Part model, mm, in its own coordinate system. A direction names the side the tool comes from. Give positions to 0.01 mm unless a question says otherwise; leave off trailing zeros. Loops run counter-clockwise (first coordinate to the right, second up) from the corner with the lowest first, then second, coordinate; pieces in that order, holes last. Notation, with made-up numbers: M -9.75,60 L 6.25,60 A14 cw 6.25,65 Z; hole C 27,-38 d6. An arc over 180 degrees is marked long. Answer in a Markdown table with one row per item.
from build123d import *

# Parameters (mm, degrees)
BOSS_EXTRUDE1_DEPTH = 20
SHELL1_T            = -2
BOSS_EXTRUDE2_START = 1
SKETCH2_R           = 50
BOSS_EXTRUDE2_DEPTH = 1
SKETCH3_R           = 2.5
CUT_EXTRUDE1_DEPTH  = 96.067235106
CIRPATTERN1_COUNT   = 3


with BuildPart() as part:
    # Sketch1 → Boss-Extrude1 (new body)
    with BuildSketch(Plane(origin=(0, 0, 0), x_dir=(1, 0, 0), z_dir=(0, 1, 0))):
        with BuildLine():
            Line((-31.353657468, -234.344603511), (-21.203657468, -216.764287814))
            Line((-21.203657468, -216.764287814), (-37.324683077, -207.456809339))
            ThreePointArc((-37.324683077, -207.456809339), (0, -190.726435625), (37.324683077, -207.456809339))
            Line((37.324683077, -207.456809339), (21.203657468, -216.764287814))
            Line((21.203657468, -216.764287814), (31.353657468, -234.344603511))
            Line((31.353657468, -234.344603511), (47.474683077, -225.037125036))
            ThreePointArc((47.474683077, -225.037125036), (43.301270189, -265.726435625), (10.15, -289.685372501))
            Line((10.15, -289.685372501), (10.15, -271.070415552))
            Line((10.15, -271.070415552), (-10.15, -271.070415552))
            Line((-10.15, -271.070415552), (-10.15, -289.685372501))
            ThreePointArc((-10.15, -289.685372501), (-43.301270189, -265.726435625), (-47.474683077, -225.037125036))
            Line((-47.474683077, -225.037125036), (-31.353657468, -234.344603511))
        make_face()
    extrude(amount=BOSS_EXTRUDE1_DEPTH)

    # Shell1
    shell1_openings = [part.faces().sort_by_distance(p)[0] for p in [
        (0, 20, 240.726435625),
        (0, 10, 190.726435625),
        (43.301270189, 10, 265.726435625),
        (-43.301270189, 10, 265.726435625),
    ]]
    offset(amount=SHELL1_T, openings=shell1_openings, kind=Kind.INTERSECTION)

    # Sketch2 → Boss-Extrude2 (add)
    with BuildSketch(Plane.XZ.offset(BOSS_EXTRUDE2_START)):
        with Locations(Location((0, 240.726435625, 0), (0, 0, 270))):
            Circle(SKETCH2_R)
    extrude(amount=-BOSS_EXTRUDE2_DEPTH)

    # Sketch3 → Cut-Extrude1 (cut, through all)
    with BuildSketch(Plane(origin=(0, 0, 269.070415552), x_dir=(-1, 0, 0), z_dir=(0, 0, -1))):
        with Locations((0, 10)):
            Circle(SKETCH3_R)
    cut_extrude1 = extrude(amount=-CUT_EXTRUDE1_DEPTH, mode=Mode.SUBTRACT)

    # CirPattern1: Cut-Extrude1 ×3 about axis
    cirpattern1_axis = Axis((0, 0, 240.726435625), (0, -1, 0))
    for i in range(1, CIRPATTERN1_COUNT):
        add(cut_extrude1.rotate(cirpattern1_axis, i * 360 / CIRPATTERN1_COUNT), mode=Mode.SUBTRACT)


solid = part.part
(1) Drill centre lines: line 1 along Y through (x, z) = (0, 270); line 2 along X through (y, z) = (14.25, 278); line 3 along Y through (x, z) = (44.5, 235.5). Where is each one in solid material? Low to high.
Recorded:
| item | result |
|---|---|
| line 1 | y = -1 to 7.5, 12.5 to 20 |
| line 2 | x = -12.15 to -10.15, 10.15 to 12.15 |
| line 3 | y = -1 to 2 |
(2) Saw through at B-B (z = 218.5). Write the cut outline in (x, y).
Recorded:
| item | result |
|---|---|
| outline | M -44.79,-1 L 44.79,-1 L 44.79,0 L 22.21,0 L 22.21,20 L 19.9,20 L 19.9,2 L -19.9,2 L -19.9,20 L -22.21,20 L -22.21,0 L -44.79,0 Z |
(3) Saw through at A-A (y = 16.75). Write the cut outline in (x, z).
Recorded:
| item | result |
|---|---|
| outline | M -48.08,227 A50 ccw -47.47,225.04 L -31.35,234.34 L -21.2,216.76 L -37.32,207.46 A50 ccw -35.93,205.95 L -18.47,216.03 L -30.62,237.08 Z; M -12.15,269.07 L 12.15,269.07 L 12.15,289.23 A50 ccw 10.15,289.69 L 10.15,271.07 L -10.15,271.07 L -10.15,289.69 A50 ccw -12.15,289.23 Z; M 18.47,216.03 L 35.93,205.95 A50 ccw 37.32,207.46 L 21.2,216.76 L 31.35,234.34 L 47.47,225.04 A50 ccw 48.08,227 L 30.62,237.08 Z |
(4) Saw through at D-D (y = 10). Give the number of separate pieces and of enclosed holes in the cut face, plus the area to 3 significant figures.
Recorded:
| item | result |
|---|---|
| separate pieces | 6 |
| enclosed holes | 0 |
| area | 337 mm^2 |
(5) Pin check, flat tips, straight feed: pin 1 Ø9.5 at (y, z) = (12.5, 282.5) entering from -X; pin 2 Ø5.5 at (y, z) = (9, 281) entering from +X; pin 3 Ø10 at (x, z) = (5, 281.5) entering from +Y; pin 4 Ø21 at (x, z) = (-30.5, 224.5) entering from +Y. Stop position of each tip, or through.
Recorded:
| item | result |
|---|---|
| pin 1 | stops at x = -12.15 |
| pin 2 | stops at x = 12.15 |
| pin 3 | stops at y = 0 |
| pin 4 | stops at y = 20 |
(6) Which spindle directions (+Z, -Z, +X, -X, +Y, -Y) get a long thin tool onto all of the face, cutting with end or side? Do faces 1 (the face through (39.301, 9.86, 229.756)), 2 (the face through (12.15, 11, 279)), 3 (the face through (0, 13, 269.07)), 4 (the face through (10.15, 10, 281)). Say none if no direction does.
Recorded:
| item | result |
|---|---|
| face 1 | +Y |
| face 2 | +Z, -Z, +X, +Y |
| face 3 | -Z, +X, -X, +Y |
| face 4 | +Z, +Y |
(7) Saw through at C-C (x = -41.5). Write the cut outline in (y, z).
Recorded:
| item | result |
|---|---|
| outline | M -1,212.84 L 0,212.84 L 0,228.49 L 20,228.49 L 20,230.8 L 2,230.8 L 2,268.61 L -1,268.61 Z |
(8) Pull direction Z, two halves, no side cores. Call faces 5 (the face through (39.228, 10.874, 232.108)), 6 (the face through (-29.151, 9.86, 212.176)), 7 (the face through (-27.08, 10.87, 211.06)): +Z half, -Z half, draft (parallel to the pull), parting line (faces both ways), or undercut.
Recorded:
| item | result |
|---|---|
| face 5 | +Z half |
| face 6 | undercut |
| face 7 | -Z half |
